```python
from build123d import *

# Parameters (mm, degrees)
F0_W     = 609.6
F0_H     = 304.8
F1_DEPTH = 1524
F2_W     = 508
F2_H     = 254
F2_H_2   = 381
F3_DEPTH = 279.4


with BuildPart() as f1:
    # F0 (on Top) → F1 (new body)
    with BuildSketch(Plane.XY):
        with Locations((-115.704429, 20.088941)):
            Rectangle(F0_W, F0_H)
    extrude(amount=F1_DEPTH)

    # F2 (on face) → F3 (cut)
    with BuildSketch(Plane.XZ.offset(132.311059)):
        with Locations((-115.704429, 1346.2)):
            Rectangle(F2_W, F2_H)
        with Locations((-115.704429, 1041.4)):
            Rectangle(F2_W, F2_H)
        with Locations((-115.704429, 673.1)):
            Rectangle(F2_W, F2_H_2)
        with Locations((-115.704429, 241.3)):
            Rectangle(F2_W, F2_H_2)
    extrude(amount=-F3_DEPTH, mode=Mode.SUBTRACT)


solid = f1.part
```
The model under review builds one solid part; all positions refer to its coordinate system, in mm. A direction names the side the tool comes from. Round coordinates to 2 decimals unless told otherwise and drop trailing zeros. Loops run counter-clockwise (first coordinate to the right, second up) from the corner with the lowest first, then second, coordinate; pieces in that order, holes last. Notation, with made-up numbers: (1, 45.5) - (28, 45.5) arc R32 cw to (28, 73.5) - close; hole circle Ø1 at (72.25, 77). An arc over 180 degrees is marked (long way). Use a Markdown table: item, result. Add a question column.
Q1. Add section A-A (x = -11). State the section outline as (y, z) points, plus the area to 3 significant figures.
Q2. Add section B-B (y = 80). State the section outline as (x, z) points.
Q3. The part is to be moulded in two halves that separate along Z. For faces 3 (the face through (138.296, 5, 239)), 4 (the face through (189.096, 18, 751)), 5 (the face through (-120, 22, 1524)), 6 (the face through (-369.704, 5, 239)), say which applies: pulls with the +Z half, pulls with the -Z half, needs draft (parallel to the pull), parting line crosses it, or undercut.
Q4. Insertion check: pin 1 Ø2 at (x, z) = (-275.5, 708) entering from -Y. The pin has a flat end and moves straight along its axis. Give the tip position at first contact, or say it passes through.
Q5. Machinability: for faces 1 (the face through (-120, 172.489, 751)), 2 (the face through (-119, 147.089, 676)), which of the approach directions +Z, -Z, +X, -X, +Y, -Y give a long, thin tool a straight path to every point of the face, cutting with its end or side? Answer none if there is none.
Q6. For probe 1 along Z at (x, y) = (121, 104); probe 2 along X at (y, z) = (-111.5, 972); probe 3 along Y at (x, z) = (80, 639.5), list the stretches that pass through material, from the lowest coordinate up.
Q7. Add section C-C (z = 532.5). State the section outline as (x, y) points, plus the area to 3 significant figures.
Worked answers:
| question | item | result |
|---|---|---|
| 1 | outline | (-132.31, 0) - (172.49, 0) - (172.49, 1524) - (-132.31, 1524) - (-132.31, 1473.2) - (147.09, 1473.2) - (147.09, 1219.2) - (-132.31, 1219.2) - (-132.31, 1168.4) - (147.09, 1168.4) - (147.09, 914.4) - (-132.31, 914.4) - (-132.31, 863.6) - (147.09, 863.6) - (147.09, 482.6) - (-132.31, 482.6) - (-132.31, 431.8) - (147.09, 431.8) - (147.09, 50.8) - (-132.31, 50.8) - close |
| 1 | area | 110,000 mm² |
| 2 | outline | (-420.5, 0) - (189.1, 0) - (189.1, 1524) - (-420.5, 1524) - close; hole (-369.7, 50.8) - (138.3, 50.8) - (138.3, 431.8) - (-369.7, 431.8) - close; hole (-369.7, 482.6) - (138.3, 482.6) - (138.3, 863.6) - (-369.7, 863.6) - close; hole (-369.7, 914.4) - (138.3, 914.4) - (138.3, 1168.4) - (-369.7, 1168.4) - close; hole (-369.7, 1219.2) - (138.3, 1219.2) - (138.3, 1473.2) - (-369.7, 1473.2) - close |
| 3 | face 3 | undercut |
| 3 | face 4 | needs draft |
| 3 | face 5 | pulls with the +Z half |
| 3 | face 6 | undercut |
| 4 | pin 1 | y = 147.09 |
| 5 | face 1 | +Z, -Z, +X, -X, +Y |
| 5 | face 2 | -Y |
| 6 | probe 1 | 0 to 50.8, 431.8 to 482.6, 863.6 to 914.4, 1168.4 to 1219.2, 1473.2 to 1524 |
| 6 | probe 2 | -420.5 to -369.7, 138.3 to 189.1 |
| 6 | probe 3 | 147.09 to 172.49 |
| 7 | outline | (-420.5, -132.31) - (-369.7, -132.31) - (-369.7, 147.09) - (138.3, 147.09) - (138.3, -132.31) - (189.1, -132.31) - (189.1, 172.49) - (-420.5, 172.49) - close |
| 7 | area | 43,900 mm² |
